Geometry: final body of the model. Coordinates: model frame, mm. Face numbers are marked on the shaded views. Give positions to 0.01 mm unless a question says otherwise; leave off trailing zeros. Write each loop counter-clockwise with the first axis right and the second up, starting at its lowest first coordinate (ties: lowest second). Pieces come first, ordered by that corner, then holes.
from build123d import *

# Parameters (mm, degrees)
SKETCH_2_R        = 2
SKETCH_2_R_2      = 1.6
EXTRUDE_3_DEPTH   = 21.5
EXTRUDE_3_2_DEPTH = 21.5
SKETCH_2_8_R      = 1.6
EXTRUDE_4_DEPTH   = 26.5
SKETCH_2_9_R      = 3
SKETCH_2_9_R_2    = 2
EXTRUDE_5_DEPTH   = 2
EXTRUDE_7_DEPTH   = 0.5
FILLET_1_R        = 0.5
SKETCH_2_12_R     = 1.6
EXTRUDE_8_DEPTH   = 25.5
FILLET_3_R        = 0.5


with BuildPart() as part:
    # Sketch 2 → Extrude 3 (new body)
    with BuildSketch(Plane.XY):
        with Locations((23.5, 37.3)):
            Circle(SKETCH_2_R)
        with Locations((23.5, 37.3)):
            Circle(SKETCH_2_R_2, mode=Mode.SUBTRACT)
    extrude(amount=EXTRUDE_3_DEPTH)

    # Sketch 2_8 → Extrude 4 (add)
    with BuildSketch(Plane.XY):
        with Locations((23.5, 37.3)):
            Circle(SKETCH_2_8_R)
    extrude(amount=EXTRUDE_4_DEPTH)

    # Sketch 2_9 → Extrude 5 (add)
    with BuildSketch(Plane.XY):
        with Locations((23.5, 37.3)):
            Circle(SKETCH_2_9_R)
        with Locations((15.2, 37.3)):
            Circle(SKETCH_2_9_R)
        with Locations((15.2, 37.3)):
            Circle(SKETCH_2_9_R_2, mode=Mode.SUBTRACT)
    extrude(amount=EXTRUDE_5_DEPTH)


with BuildPart() as body_2:
    # Sketch 2 → Extrude 3 2 (new body)
    with BuildSketch(Plane.XY):
        with Locations((15.2, 37.3)):
            Circle(SKETCH_2_R)
        with Locations((15.2, 37.3)):
            Circle(SKETCH_2_R_2, mode=Mode.SUBTRACT)
    extrude(amount=EXTRUDE_3_2_DEPTH)


with BuildPart() as extrude_5_piece_1:
    # of the separate pieces the step leaves, piece 1, a body of its own (extrude_5_pieces)
    add(part.part.solids().sort_by_distance((26.5, 37.3, 0))[0])

    # Sketch 2_11 → Extrude 7 (add)
    with BuildSketch(Plane.XY):
        with BuildLine():
            ThreePointArc((17.239607805, 35.1), (16.295445115, 34.507151991), (15.2, 34.3))
            Line((15.2, 34.3), (23.5, 34.3))
            ThreePointArc((23.5, 34.3), (22.404554885, 34.507151991), (21.460392195, 35.1))
            Line((21.460392195, 35.1), (17.239607805, 35.1))
        make_face()
        with BuildLine():
            Line((23.5, 40.3), (15.2, 40.3))
            ThreePointArc((15.2, 40.3), (16.295445115, 40.092848009), (17.239607805, 39.5))
            Line((17.239607805, 39.5), (21.460392195, 39.5))
            ThreePointArc((21.460392195, 39.5), (22.404554885, 40.092848009), (23.5, 40.3))
        make_face()
    extrude(amount=EXTRUDE_7_DEPTH)

    # Fillet 1
    fillet_1_edges = [extrude_5_piece_1.edges().sort_by_distance(p)[0] for p in [
        (21.9, 37.3, 26.5),
    ]]
    fillet(fillet_1_edges, radius=FILLET_1_R)



with BuildPart() as extrude_5_piece_2:
    # of the separate pieces the step leaves, piece 2, a body of its own (extrude_5_pieces)
    add(part.part.solids().sort_by_distance((18.2, 37.3, 0))[0])


with BuildPart() as extrude_5_piece_1_1:
    add(extrude_5_piece_1.part)

    add(extrude_5_piece_2.part)  # Extrude 8 merges Extrude 5 piece 2

    add(body_2.part)  # Extrude 8 merges body 2
    # Sketch 2_12 → Extrude 8 (add)
    with BuildSketch(Plane.XY):
        with Locations((15.2, 37.3)):
            Circle(SKETCH_2_12_R)
    extrude(amount=EXTRUDE_8_DEPTH)

    # Fillet 3
    fillet_3_edges = [extrude_5_piece_1_1.edges().sort_by_distance(p)[0] for p in [
        (13.6, 37.3, 25.5),
    ]]
    fillet(fillet_3_edges, radius=FILLET_3_R)


solid = extrude_5_piece_1_1.part
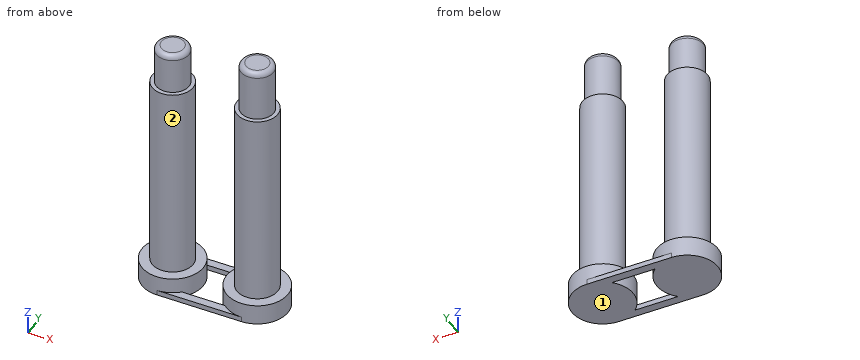
Q1. Section D-D on y = 39.8. Output: boundary loops of the cut face in (x, z).
Filled sheet:
outline: (13.54, 0) - (25.16, 0) - (25.16, 2) - (21.84, 2) - (21.84, 0.5) - (16.86, 0.5) - (16.86, 2) - (13.54, 2) - close
Q2. Pull-direction query (X, two-part tool) for the marked faces 1 and 2; classes: released by +X, released by -X, zero draft, split by the parting line, or undercut.
Filled sheet:
face 1: zero draft
face 2: undercut
Q3. Section A-A on y = 37.3. Output: boundary loops of the cut face in (x, z), plus the area to 3 significant figures.
Filled sheet:
outline: (12.2, 0) - (18.2, 0) - (18.2, 2) - (17.2, 2) - (17.2, 21.5) - (16.8, 21.5) - (16.8, 25) arc R0.5 ccw to (16.3, 25.5) - (14.1, 25.5) arc R0.5 ccw to (13.6, 25) - (13.6, 21.5) - (13.2, 21.5) - (13.2, 2) - (12.2, 2) - close; (20.5, 0) - (26.5, 0) - (26.5, 2) - (25.5, 2) - (25.5, 21.5) - (25.1, 21.5) - (25.1, 26) arc R0.5 ccw to (24.6, 26.5) - (22.4, 26.5) arc R0.5 ccw to (21.9, 26) - (21.9, 21.5) - (21.5, 21.5) - (21.5, 2) - (20.5, 2) - close
area: 209 mm2
Q4. Pin query (flat end, axial travel): P1, Ø0.6, axis at x = 17.5, y = 40, coming from the +Z side; P2, Ø1, axis at x = 21, y = 36, coming from the +Z side; P3, Ø1.8, axis at x = 16, y = 37.5, coming from the +Z side. Return the tip coordinate at first contact, or that it passes through.
Filled sheet:
P1: stops at z = 0.5
P2: stops at z = 2
P3: stops at z = 25.5
Q5. Ray query, line 1 along X through (y, z) = (37.2, 19.5); line 2 along Z through (x, y) = (25, 36.4); line 3 along Z through (x, y) = (17.25, 35). Return the intervals inside material, ascending.
Filled sheet:
line 1: x = 13.2 to 17.2, 21.5 to 25.5
line 2: z = 0 to 21.5
line 3: z = 0 to 0.5
Q6. Section C-C on z = 12.25. Output: boundary loops of the cut face in (x, y), plus the area to 3 significant figures.
Filled sheet:
outline: circle Ø4 at (15.2, 37.3); circle Ø4 at (23.5, 37.3)
area: 25.1 mm2
Q7. Section B-B on x = 18.5. Output: boundary loops of the cut face in (y, z), plus the area to 3 significant figures.
Filled sheet:
outline: (34.3, 0) - (35.1, 0) - (35.1, 0.5) - (34.3, 0.5) - close; (39.5, 0) - (40.3, 0) - (40.3, 0.5) - (39.5, 0.5) - close
area: 0.800 mm2
